Can you work these out from the model? Positions are in its coordinate system, mm. Round coordinates to 2 decimals unless told otherwise and drop trailing zeros. Order: outer loops, then holes, each group sorted by start corner. A loop starts at its lowest first (then second) coordinate and runs counter-clockwise, first axis right, second up. Notation, with made-up numbers: (67.5, -2.75) -> (95.5, -2.75) arc R3 ccw to (95.5, 2.25) -> close; hole circle Ø3 at (-5.75, 68.25). An arc over 180 degrees is marked (long way). One line per item, written item: value.
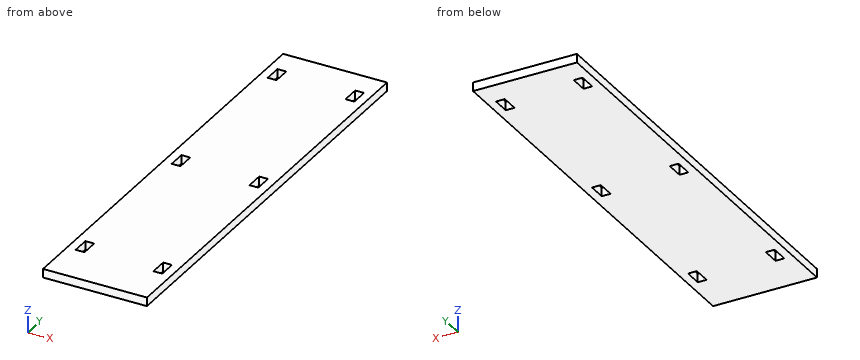
Autodesk Inventor part; units mm, degrees
ref_plane "YZ Plane" through (0, 0, 0) normal (1, 0, 0) x (0, 1, 0)
ref_plane "XZ Plane" through (0, 0, 0) normal (0, 1, 0) x (-1, 0, 0)
ref_plane "XY Plane" through (0, 0, 0) normal (0, 0, 1) x (1, 0, 0)
sketch "Sketch1" plane through (0, 0, 0) normal (0, 0, 1) x (1, 0, 0)
  line L0 (-1.9934, -116.9491) -> (8.0066, -116.9491) construction
  line L1 (38.0066, 133.0509) -> (38.0066, -116.9491) construction
  line L2 (8.0066, 133.0509) -> (8.0066, -116.9491)
  line L3 (63.0066, 8.0509) -> (63.0066, -81.8491) construction
  line L4 (57.9066, 8.0509) -> (57.9066, -81.8491) construction
  line L5 (8.0066, -116.9491) -> (68.0066, -116.9491)
  line L6 (57.9066, -91.9491) -> (63.0066, -91.9491)
  line L7 (63.0066, -81.8491) -> (57.9066, -81.8491)
  line L8 (68.0066, 133.0509) -> (8.0066, 133.0509)
  line L9 (57.9066, 18.1509) -> (57.9066, 8.0509)
  line L10 (57.9066, 8.0509) -> (63.0066, 8.0509)
  line L11 (18.1066, 18.1509) -> (18.1066, 8.0509)
  line L12 (13.0066, 18.1509) -> (13.0066, 8.0509)
  line L13 (18.1066, 8.0509) -> (13.0066, 8.0509)
  line L14 (63.0066, 18.1509) -> (63.0066, 8.0509)
  line L15 (18.1066, 18.1509) -> (13.0066, 18.1509)
  line L16 (73.0066, 108.0509) -> (8.0066, 108.0509) construction
  line L17 (73.0066, 118.1509) -> (8.0066, 118.1509) construction
  line L18 (63.0066, 118.1509) -> (63.0066, 108.0509)
  line L19 (57.9066, 118.1509) -> (57.9066, 108.0509)
  line L20 (63.0066, 118.1509) -> (57.9066, 118.1509)
  line L21 (57.9066, 108.0509) -> (63.0066, 108.0509)
  line L22 (57.9066, 108.0509) -> (57.9066, 18.1509) construction
  line L23 (63.0066, 108.0509) -> (63.0066, 18.1509) construction
  line L24 (57.9066, 18.1509) -> (63.0066, 18.1509)
  line L25 (57.9066, -81.8491) -> (57.9066, -91.9491)
  line L26 (63.0066, -81.8491) -> (63.0066, -91.9491)
  line L27 (13.0066, -81.8491) -> (18.1066, -81.8491)
  line L28 (13.0066, -81.8491) -> (13.0066, -91.9491)
  line L29 (18.1066, -81.8491) -> (18.1066, -91.9491)
  line L30 (18.1066, -91.9491) -> (13.0066, -91.9491)
  line L31 (-1.9934, -91.9491) -> (68.0066, -91.9491) construction
  line L32 (8.0066, -116.9491) -> (-1.9934, -116.9491) construction
  line L33 (-1.9934, -81.8491) -> (68.0066, -81.8491) construction
  line L34 (3.0066, 108.0509) -> (68.0066, 108.0509) construction
  line L35 (3.0066, 118.1509) -> (68.0066, 118.1509) construction
  line L36 (18.1066, 108.0509) -> (13.0066, 108.0509)
  line L37 (13.0066, 118.1509) -> (13.0066, 108.0509)
  line L38 (13.0066, 118.1509) -> (18.1066, 118.1509)
  line L39 (18.1066, 118.1509) -> (18.1066, 108.0509)
  line L40 (68.0066, -116.9491) -> (68.0066, 133.0509)
  point P0 (0, 0)
extrude "Extrusion1" add sketch "Sketch1" along normal blind 5
properties part number "Lifting Sections right"
Q1. Will this pin go through, and if not, where does the flat tip stop? pin 1 Ø12 at (x, y) = (53.5, -68) entering from -Z.
Answers below:
pin 1: z = 0
Q2. I want a section at A-A on y = 110.5. List the corners of the cut face in (x, z) for me, plus the area to 3 significant figures.
Answers below:
outline: (8.01, 0) -> (13.01, 0) -> (13.01, 5) -> (8.01, 5) -> close; (18.11, 0) -> (57.91, 0) -> (57.91, 5) -> (18.11, 5) -> close; (63.01, 0) -> (68.01, 0) -> (68.01, 5) -> (63.01, 5) -> close
area: 249 mm^2
Q3. Please list where these lines run through material, in increasing order: line 1 along X through (y, z) = (-87.5, 1.7); line 2 along Y through (x, z) = (17.5, 1.3).
Answers below:
line 1: 8.01 to 13.01, 18.11 to 57.91, 63.01 to 68.01
line 2: -116.95 to -91.95, -81.85 to 8.05, 18.15 to 108.05, 118.15 to 133.05
Q4. I want a section at B-B on z = 0.8. List the corners of the cut face in (x, y) for me, plus the area to 3 significant figures.
Answers below:
outline: (8.01, -116.95) -> (68.01, -116.95) -> (68.01, 133.05) -> (8.01, 133.05) -> close; hole (13.01, -91.95) -> (18.11, -91.95) -> (18.11, -81.85) -> (13.01, -81.85) -> close; hole (13.01, 8.05) -> (18.11, 8.05) -> (18.11, 18.15) -> (13.01, 18.15) -> close; hole (13.01, 108.05) -> (18.11, 108.05) -> (18.11, 118.15) -> (13.01, 118.15) -> close; hole (57.91, -91.95) -> (63.01, -91.95) -> (63.01, -81.85) -> (57.91, -81.85) -> close; hole (57.91, 8.05) -> (63.01, 8.05) -> (63.01, 18.15) -> (57.91, 18.15) -> close; hole (57.91, 108.05) -> (63.01, 108.05) -> (63.01, 118.15) -> (57.91, 118.15) -> close
area: 14,700 mm^2
